Work out the finished part from the listing and answer in its coordinate system (mm). A direction names the side the tool comes from. Give positions to 0.01 mm unless a question says otherwise; leave off trailing zeros. Order: outer loops, then holes, each group sorted by start corner. A loop starts at its lowest first (then second) coordinate and runs counter-clockwise, first axis right, second up.
```python
from build123d import *

# Parameters (mm, degrees)
CROQUIS1_W              = 97.7
CROQUIS1_H              = 85
CROQUIS1_R              = 3
CROQUIS1_R_2            = 30
SALIENTE_EXTRUIR1_DEPTH = 10
CROQUIS2_R              = 5
SALIENTE_EXTRUIR2_DEPTH = 350
CROQUIS3_W              = 97.7
CROQUIS3_H              = 85
SALIENTE_EXTRUIR3_DEPTH = 20
CHAFL_N1_SIZE           = 1


with BuildPart() as part:
    # Croquis1 → Saliente-Extruir1 (new body)
    with BuildSketch(Plane.XY):
        Rectangle(CROQUIS1_W, CROQUIS1_H)
        with Locations((-34.85, 36.5)):
            Circle(CROQUIS1_R, mode=Mode.SUBTRACT)
        Circle(CROQUIS1_R_2, mode=Mode.SUBTRACT)
        with Locations(Location((34.85, 36.5, 0), (0, 0, 180))):
            Circle(CROQUIS1_R, mode=Mode.SUBTRACT)
        with Locations((34.85, -36.5)):
            Circle(CROQUIS1_R, mode=Mode.SUBTRACT)
        with Locations(Location((-34.85, -36.5, 0), (0, 0, 180))):
            Circle(CROQUIS1_R, mode=Mode.SUBTRACT)
    extrude(amount=SALIENTE_EXTRUIR1_DEPTH)

    # Croquis2 → Saliente-Extruir2 (add)
    with BuildSketch(Plane.XY.offset(10)):
        with Locations((-40, 0)):
            Circle(CROQUIS2_R)
        with Locations(Location((40, 0, 0), (0, 0, 180))):
            Circle(CROQUIS2_R)
    extrude(amount=SALIENTE_EXTRUIR2_DEPTH)

    # Croquis3 → Saliente-Extruir3 (add)
    with BuildSketch(Plane.XY.offset(360)):
        Rectangle(CROQUIS3_W, CROQUIS3_H)
    extrude(amount=SALIENTE_EXTRUIR3_DEPTH)

    # Chaflán1
    chafl_n1_edges = [part.edges().sort_by_distance(p)[0] for p in [
        (48.85, 0, 10),
        (0, 42.5, 10),
        (-48.85, 0, 360),
        (-48.85, 42.5, 370),
        (48.85, 0, 360),
        (0, 42.5, 360),
        (48.85, 42.5, 370),
        (-48.85, 0, 10),
        (-48.85, 42.5, 5),
        (48.85, 42.5, 5),
    ]]
    chamfer(chafl_n1_edges, length=CHAFL_N1_SIZE)


solid = part.part
```
1. The mould has two halves that part along Z. Classify faces 4 (the face through (-11.3, 28.1, 10)), 5 (the face through (-1, 42.5, 370)), 6 (the face through (-1, 1, 380)): pulls with the +Z half, pulls with the -Z half, needs draft (parallel to the pull), parting line crosses it, or undercut.
Findings below:
face 4: undercut
face 5: needs draft
face 6: pulls with the +Z half
2. The part is cut by section D-D (x = 0). Write down the section's boundary in (y, z).
Findings below:
outline: (-42.5, 0) - (-30, 0) - (-30, 10) - (-42.5, 10) - close; (-42.5, 360) - (41.5, 360) - (42.5, 361) - (42.5, 380) - (-42.5, 380) - close; (30, 0) - (42.5, 0) - (42.5, 9) - (41.5, 10) - (30, 10) - close
3. Straight lines are drawn through the part: probe 1 along Y at (x, z) = (-34.85, 4.5); probe 2 along X at (y, z) = (-36, 3); probe 3 along Z at (x, y) = (39, -13.5). For each, find the intervals that lie inside material, in ascending order.
Findings below:
probe 1: y = -42.5 to -39.5, -33.5 to 33.5, 39.5 to 42.5
probe 2: x = -48.85 to -37.81, -31.89 to 31.89, 37.81 to 48.85
probe 3: z = 0 to 10, 360 to 380
4. The part is cut by section B-B (y = 8.5). Write down the section's boundary in (x, z).
Findings below:
outline: (-48.85, 0) - (-28.77, 0) - (-28.77, 10) - (-47.85, 10) - (-48.85, 9) - close; (-48.85, 361) - (-47.85, 360) - (47.85, 360) - (48.85, 361) - (48.85, 380) - (-48.85, 380) - close; (28.77, 0) - (48.85, 0) - (48.85, 9) - (47.85, 10) - (28.77, 10) - close
5. The part is cut by section A-A (x = 24). Write down the section's boundary in (y, z), then the cut area to 3 significant figures.
Findings below:
outline: (-42.5, 0) - (-18, 0) - (-18, 10) - (-42.5, 10) - close; (-42.5, 360) - (41.5, 360) - (42.5, 361) - (42.5, 380) - (-42.5, 380) - close; (18, 0) - (42.5, 0) - (42.5, 9) - (41.5, 10) - (18, 10) - close
area: 2,190 mm2
6. Given P1, Ø5, axis at x = 36.5, z = 316, coming from the +Y side; P2, Ø8, axis at x = -34.85, y = -36.5, coming from the -Z side; P3, Ø3, axis at y = -3, z = 163, coming from the +X side, each flat-ended and moving along its own axis, determine where each tip first touches the part or whether it passes through.
Findings below:
P1: stops at y = 4.9
P2: stops at z = 0
P3: stops at x = 44.77
7. Which of the six approach directions +Z, -Z, +X, -X, +Y, -Y give full straight-line access (tool end or side, diameter ignored) to faces 1 (the face through (48.85, -1, 370)), 2 (the face through (45, 0, 183)), 3 (the face through (-29.97, 1.32, 4.93))?
Findings below:
face 1: +Z, -Z, +X, +Y, -Y
face 2: none
face 3: -Z
8. The part is cut by section C-C (z = 27). Write down the section's boundary in (x, y), then the cut area to 3 significant figures.
Findings below:
outline: circle Ø10 at (-40, 0); circle Ø10 at (40, 0)
area: 157 mm2
